Read the model definition and answer for the solid it produces. Units are mm, in the model's axes. Face numbers are marked on the shaded views. Coordinates: 2 decimals unless noted, no trailing zeros. Write each loop counter-clockwise with the first axis right and the second up, starting at its lowest first coordinate (ties: lowest second). Pieces come first, ordered by that corner, then holes.
1) The part is cut by section A-A (x = -15). Determine the outline of the cut face in (y, z).
2) The part is cut by section B-B (y = 2.3). Give the number of separate pieces and of enclosed holes in the cut face, then the cut area to 3 significant figures.
3) Determine the mould class of the marked faces 1 and 2 for opening direction X: +X half, -X half, draft (parallel to the pull), parting line (faces both ways), or undercut.
4) Find the intervals of material crossed by line 1 (Z direction, x = 27, y = 2.25); line 2 (Z direction, x = -3, y = 1.65); line 3 (Z direction, x = -35, y = 2.5), in increasing order.
5) This flat-tipped pin is pushed along its axis until it touches: pin 1 Ø4.5 at (x, z) = (25, 3) entering from +Y. Where does it stop, or does it pass through?
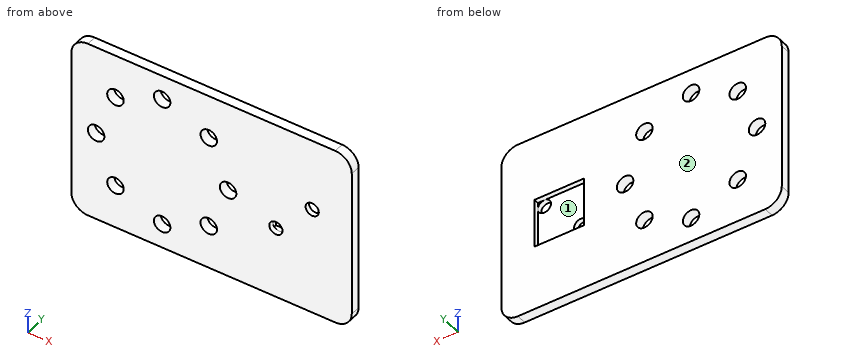
from build123d import *

# Parameters (mm, degrees)
SKETCH1_W           = 85
SKETCH1_H           = 55
SKETCH1_R           = 2.5
SKETCH1_W_2         = 15
SKETCH1_H_2         = 15
BOSS_EXTRUDE3_DEPTH = 3
FILLET2_R           = 5
BOSS_EXTRUDE4_REACH = 27
SKETCH2_W           = 15
SKETCH2_H           = 1.5
SKETCH3_R           = 2
CUT_EXTRUDE1_DEPTH  = 10


with BuildPart() as part:
    # Sketch1 → Boss-Extrude3 (new body)
    with BuildSketch(Plane(origin=(0, 0, 0), x_dir=(1, 0, 0), z_dir=(0, 1, 0))):
        with Locations((0, -0.433266932)):
            Rectangle(SKETCH1_W, SKETCH1_H)
        with Locations((-35, -0.433266932)):
            Circle(SKETCH1_R, mode=Mode.SUBTRACT)
        with Locations((-29.142135624, 13.708868691)):
            Circle(SKETCH1_R, mode=Mode.SUBTRACT)
        with Locations((-15, 19.566733068)):
            Circle(SKETCH1_R, mode=Mode.SUBTRACT)
        with Locations((-0.857864376, 13.708868691)):
            Circle(SKETCH1_R, mode=Mode.SUBTRACT)
        with Locations((5, -0.433266932)):
            Circle(SKETCH1_R, mode=Mode.SUBTRACT)
        with Locations((-0.857864376, -14.575402556)):
            Circle(SKETCH1_R, mode=Mode.SUBTRACT)
        with Locations((-15, -20.433266932)):
            Circle(SKETCH1_R, mode=Mode.SUBTRACT)
        with Locations((-29.142135624, -14.575402556)):
            Circle(SKETCH1_R, mode=Mode.SUBTRACT)
        with Locations((25, -0.433266932)):
            Rectangle(SKETCH1_W_2, SKETCH1_H_2, mode=Mode.SUBTRACT)
    extrude(amount=BOSS_EXTRUDE3_DEPTH)

    # Fillet2
    fillet2_edges = [part.edges().sort_by_distance(p)[0] for p in [
        (42.5, 1.5, 27.933266932),
        (-42.5, 1.5, 27.933266932),
        (-42.5, 1.5, -27.066733068),
        (42.5, 1.5, -27.066733068),
    ]]
    fillet(fillet2_edges, radius=FILLET2_R)

    # Sketch2 → Boss-Extrude4 (add, up to next)
    with BuildSketch(Plane(origin=(17.5, 0, 0), x_dir=(0, 0, -1), z_dir=(1, 0, 0)), mode=Mode.PRIVATE) as boss_extrude4_sk1:
        with Locations((-0.433266932, 0.75)):
            Rectangle(SKETCH2_W, SKETCH2_H)
    boss_extrude4_tool1 = extrude(boss_extrude4_sk1.sketch, amount=BOSS_EXTRUDE4_REACH, mode=Mode.PRIVATE) - part.part
    add(boss_extrude4_tool1.solids().sort_by_distance((17.5, 0.75, 0.433267))[0])

    # Sketch3 → Cut-Extrude1 (cut)
    with BuildSketch(Plane(origin=(0, 1.5, 0), x_dir=(1, 0, 0), z_dir=(0, 1, 0))):
        with Locations((30.5, -5.933266932)):
            Circle(SKETCH3_R)
        with Locations((19.5, 5.066733068)):
            Circle(SKETCH3_R)
    extrude(amount=-CUT_EXTRUDE1_DEPTH, mode=Mode.SUBTRACT)


solid = part.part
Reported:
1. outline: (0, -27.07) - (3, -27.07) - (3, -22.07) - (0, -22.07) - close; (0, -17.07) - (3, -17.07) - (3, 17.93) - (0, 17.93) - close; (0, 22.93) - (3, 22.93) - (3, 27.93) - (0, 27.93) - close
2. separate pieces: 1
2. enclosed holes: 9
2. area: 4,270 mm2
3. face 1: undercut
3. face 2: draft
4. line 1: z = -27.07 to -7.07, 7.93 to 27.93
4. line 2: z = -27.07 to -15, -12.42 to 13.29, 15.86 to 27.93
4. line 3: z = -27.07 to -2.07, 2.93 to 27.93
5. pin 1: stops at y = 1.5
